Check sheet for the modelled part. Datum: model origin and axes. Units: mm. Give positions to 0.01 mm unless a question says otherwise; leave off trailing zeros. Write each loop counter-clockwise with the first axis right and the second up, starting at its lowest first coordinate (ties: lowest second). Pieces come first, ordered by that corner, then holes. Notation, with made-up numbers: (-16.5, 75) -> (10.5, 75) arc R24 cw to (10.5, 93) -> close; hole circle Ø3 at (42.25, 66). An arc over 180 degrees is marked (long way). Use a Markdown table: item, result. Add a question column.
1. Release check for a two-part mould opening along X. For faces 1 (the flat face through (7.698, -13, 5)), 2 (the flat face through (21, 10.101, 5)), 3 (the flat face through (33.098, -3, 5)) record: released by +X, released by -X, zero draft, split by the parting line, or undercut.
2. Scan lines: probe 1 along Y at (x, z) = (25.5, 6.75); probe 2 along X at (y, z) = (-13, 7); probe 3 along X at (y, z) = (0.5, 1.5). Record each from-to range of solid material in increasing order. Write a range as [from, to].
3. Cross-section at B-B (y = -11.75). Enter the section's corners in (x, z), then the cut area to 3 significant figures.
4. Cross-section at C-C (x = 0). Enter the section's corners in (y, z).
5. Gauge pin test, flat ends, axial feed: P1, Ø4, axis at x = -4.5, y = -9, coming from the -Z side; P2, Ø1.6, axis at y = -11.5, z = 5.5, coming from the -X side; P3, Ø1.5, axis at x = 25.5, z = 6, coming from the +Y side; P4, Ø2, axis at x = -1.5, z = 5.5, coming from the -Y side. Record the tip position at first contact, or that the pin passes through.
6. Cross-section at A-A (z = 2.5). Enter the section's corners in (x, y).
from build123d import *

# Parameters (mm, degrees)
F1_DEPTH = 10


with BuildPart() as f1:
    # F0 (on Top) → F1 (new body)
    with BuildSketch(Plane.XY):
        with BuildLine():
            ThreePointArc((7.6980242142, -10.1010109988), (11.3810128618, -5.6358270236), (12.7, 0))
            ThreePointArc((12.7, 0), (11.3810128618, 5.6358270236), (7.6980242142, 10.1010109988))
            Line((7.6980242142, 10.1010109988), (7.6980242142, -10.1010109988))
        make_face()
        with BuildLine():
            ThreePointArc((7.6980242142, 10.1010109988), (11.3810128618, 5.6358270236), (12.7, 0))
            ThreePointArc((12.7, 0), (11.3810128618, -5.6358270236), (7.6980242142, -10.1010109988))
            Line((7.6980242142, -10.1010109988), (7.6980242142, -15.2989890012))
            Line((7.6980242142, -15.2989890012), (33.0980242142, -15.2989890012))
            Line((33.0980242142, -15.2989890012), (33.0980242142, 10.1010109988))
            Line((33.0980242142, 10.1010109988), (7.6980242142, 10.1010109988))
        make_face()
        with BuildLine():
            Line((7.6980242142, -10.1010109988), (7.6980242142, 10.1010109988))
            ThreePointArc((7.6980242142, 10.1010109988), (-12.7, 0), (7.6980242142, -10.1010109988))
        make_face()
    extrude(amount=F1_DEPTH)


solid = f1.part
Worked answers:
| question | item | result |
|---|---|---|
| 1 | face 1 | undercut |
| 1 | face 2 | zero draft |
| 1 | face 3 | released by +X |
| 2 | probe 1 | y = [-15.3, 10.1] |
| 2 | probe 2 | x = [7.7, 33.1] |
| 2 | probe 3 | x = [-12.69, 33.1] |
| 3 | outline | (-4.82, 0) -> (4.82, 0) -> (4.82, 10) -> (-4.82, 10) -> close; (7.7, 0) -> (33.1, 0) -> (33.1, 10) -> (7.7, 10) -> close |
| 3 | area | 350 mm² |
| 4 | outline | (-12.7, 0) -> (12.7, 0) -> (12.7, 10) -> (-12.7, 10) -> close |
| 5 | P1 | stops at z = 0 |
| 5 | P2 | stops at x = -6.84 |
| 5 | P3 | stops at y = 10.1 |
| 5 | P4 | stops at y = -12.69 |
| 6 | outline | (7.7, -15.3) -> (33.1, -15.3) -> (33.1, 10.1) -> (7.7, 10.1) arc R12.7 ccw (long way) to (7.7, -10.1) -> close |
